Check sheet for the modelled part. Datum: model origin and axes. Units: mm. Face numbers are marked on the shaded views. A direction names the side the tool comes from. Round coordinates to 2 decimals unless told otherwise and drop trailing zeros. Order: outer loops, then holes, each group sorted by start corner. A loop starts at its lowest first (then second) coordinate and runs counter-clockwise, first axis right, second up. Notation, with made-up numbers: (31.25, -7) -> (71.25, -7) arc R14 ccw to (71.25, -3) -> close; hole circle Ø10 at (-19, 4.25). An arc over 180 degrees is marked (long way). Answer in a Markdown table with one row per item.
```python
from build123d import *

# Parameters (mm, degrees)
SKETCH1_W           = 18
SKETCH1_H           = 10.5
SKETCH1_R           = 1.625
BOSS_EXTRUDE1_DEPTH = 1
SKETCH2_W           = 18
SKETCH2_H           = 1
BOSS_EXTRUDE2_DEPTH = 9
SKETCH4_R           = 1.625
CUT_EXTRUDE1_DEPTH  = 23.677080941


with BuildPart() as part:
    # Sketch1 → Boss-Extrude1 (new body)
    with BuildSketch(Plane(origin=(0, 0, 0), x_dir=(1, 0, 0), z_dir=(0, 1, 0))):
        with Locations((9, 5.25)):
            Rectangle(SKETCH1_W, SKETCH1_H)
        with Locations(Location((6, 3, 0), (0, 0, 270))):
            Circle(SKETCH1_R, mode=Mode.SUBTRACT)
        with Locations(Location((12, 3, 0), (0, 0, 270))):
            Circle(SKETCH1_R, mode=Mode.SUBTRACT)
    extrude(amount=BOSS_EXTRUDE1_DEPTH)

    # Sketch2 → Boss-Extrude2 (add)
    with BuildSketch(Plane(origin=(0, 1, 0), x_dir=(1, 0, 0), z_dir=(0, 1, 0))):
        with Locations((9, 10)):
            Rectangle(SKETCH2_W, SKETCH2_H)
    extrude(amount=BOSS_EXTRUDE2_DEPTH)

    # Sketch4 → Cut-Extrude1 (cut, through all)
    with BuildSketch(Plane.XY.offset(-9.5)):
        with Locations((6, 7)):
            Circle(SKETCH4_R)
        with Locations((12, 7)):
            Circle(SKETCH4_R)
    extrude(amount=-CUT_EXTRUDE1_DEPTH, mode=Mode.SUBTRACT)


solid = part.part
```
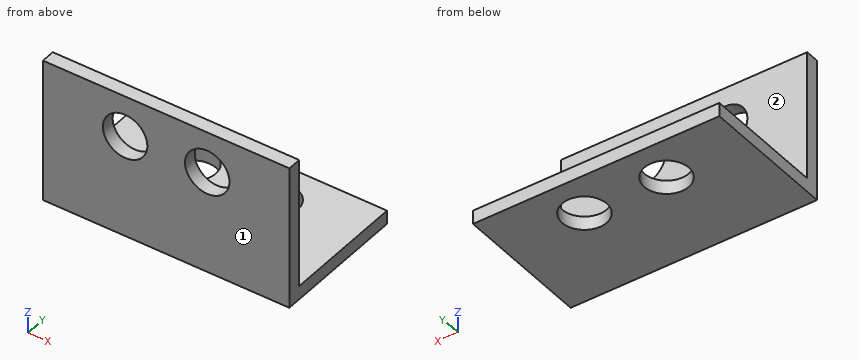
(1) Section check B-B on z = -3. Record the boundary of the cut face in (x, y) (3 decimals), plus the area to 3 significant figures.
Solutions:
| item | result |
|---|---|
| outline | (0, 0) -> (4.375, 0) -> (4.375, 1) -> (0, 1) -> close; (7.625, 0) -> (10.375, 0) -> (10.375, 1) -> (7.625, 1) -> close; (13.625, 0) -> (18, 0) -> (18, 1) -> (13.625, 1) -> close |
| area | 11.5 mm^2 |
(2) Tool access check on the marked faces 1 and 2. Record the directions out of +Z, -Z, +X, -X, +Y, -Y that give a thin tool (end or side, any length) a straight path to the whole face; none if there is none.
Solutions:
| item | result |
|---|---|
| face 1 | +Z, -Z, +X, -X, -Y |
| face 2 | +Z, +X, -X, +Y |
(3) Section check C-C on x = 9. Record the boundary of the cut face in (y, z).
Solutions:
| item | result |
|---|---|
| outline | (0, -10.5) -> (10, -10.5) -> (10, -9.5) -> (1, -9.5) -> (1, 0) -> (0, 0) -> close |
(4) Section check A-A on x = 12. Record the boundary of the cut face in (y, z) (3 decimals), plus the area to 3 significant figures.
Solutions:
| item | result |
|---|---|
| outline | (0, -10.5) -> (5.375, -10.5) -> (5.375, -9.5) -> (1, -9.5) -> (1, -4.625) -> (0, -4.625) -> close; (0, -1.375) -> (1, -1.375) -> (1, 0) -> (0, 0) -> close; (8.625, -10.5) -> (10, -10.5) -> (10, -9.5) -> (8.625, -9.5) -> close |
| area | 13.0 mm^2 |
(5) Section check D-D on z = -4.25. Record the boundary of the cut face in (x, y), plus the area to 3 significant figures.
Solutions:
| item | result |
|---|---|
| outline | (0, 0) -> (4.96, 0) -> (4.96, 1) -> (0, 1) -> close; (7.04, 0) -> (10.96, 0) -> (10.96, 1) -> (7.04, 1) -> close; (13.04, 0) -> (18, 0) -> (18, 1) -> (13.04, 1) -> close |
| area | 13.8 mm^2 |
(6) Scan lines: probe 1 along X at (y, z) = (0.45, -3) (3 decimals); probe 2 along Y at (x, z) = (12, -9.65) (3 decimals); probe 3 along Y at (x, z) = (6.25, -8). Record each from-to range of solid material in increasing order. Write a range as from..to.
Solutions:
| item | result |
|---|---|
| probe 1 | 0..4.375, 7.625..10.375, 13.625..18 |
| probe 2 | 0..5.375, 8.625..10 |
| probe 3 | 0..1 |
(7) Depth check by flat-ended pin: pin 1 Ø1.9 at (x, y) = (6, 7) entering from +Z (1 decimal); pin 2 Ø1.5 at (x, z) = (16, -7.5) entering from +Y. Enter the tip coordinate at first touch or a pass-through.
Solutions:
| item | result |
|---|---|
| pin 1 | through |
| pin 2 | y = 1 |
